Part model, mm, in its own coordinate system. A direction names the side the tool comes from. Coordinates: 2 decimals unless noted, no trailing zeros. Loops run counter-clockwise (first coordinate to the right, second up) from the corner with the lowest first, then second, coordinate; pieces in that order, holes last. Notation, with made-up numbers: M 61.25,25.25 L 110.25,25.25 A21 ccw 110.25,59.25 Z; hole C 87,56.5 d4. An arc over 180 degrees is marked long. Answer as a JSON object with one key per item and string values. Group by question number.
1. Saw through at C-C on y = -12. Write the cut outline in (x, z).
2. Saw through at A-A on x = 0. Write the cut outline in (y, z), then the cut area to 3 significant figures.
3. Saw through at D-D on x = -4.5. Write the cut outline in (y, z).
4. Drop flat-ended pins along their axis: pin 1 Ø3 at (x, y) = (-2.5, 6.5) entering from -Z; pin 2 Ø3 at (x, z) = (-7.5, 0) entering from +Y; pin 3 Ø5 at (x, y) = (-3, -13) entering from +Z; pin 4 Ø7.5 at (x, z) = (3, 1.5) entering from -Y. Give the stop position or say it passes through.
5. Drill centre lines: L1, parallel to X at y = -1.35, z = 0; L2, parallel to Z at x = 7.5, y = -2.6; L3, parallel to Y at x = 6.5, z = 2. Where is each one in solid material? Low to high.
6. Mould opens along Z. For faces 1 (the face through (0, -31, 7.7)), 2 (the face through (0, 10, 2)), 3 (the face through (7, -5, 0)) say: released by +Z, released by -Z, zero draft, split by the parting line, or undercut.
7. 3-axis set-ups, long thin cutter, end or side, ignore diameter. For faces 4 (the face through (-7.66, -45.87, -1.51)), 5 (the face through (-8, -5, 0)), 6 (the face through (7.53, -45.875, 1.783)), 7 (the face through (-7.53, -45.875, -1.783)), 8 (the face through (0, -19, -9)): which of +Z, -Z, +X, -X, +Y, -Y reach the whole face in a straight line?
from build123d import *

# Parameters (mm, degrees)
SKETCH_R                 = 10
PAD_DEPTH                = 19
SKETCH001_R              = 3.5
PAD001_DEPTH             = 3
SKETCH002_R              = 2
PAD002_DEPTH             = 14.5
SKETCH003_W              = 10
SKETCH003_H              = 5
POCKET_DEPTH             = 14.5
PAD003_DEPTH             = 25.1
SKETCH005_R              = 3.1
PAD004_DEPTH             = 2.1
SKETCH006_R              = 1
PAD005_DEPTH             = 6
PAD006_DEPTH             = 3.6
SKETCH009_R              = 0.5
POCKET001_DEPTH          = 5
POLARPATTERN_COUNT       = 2
POLARPATTERN001_COUNT    = 2
POLARPATTERN001_FACE35_R = 1
POCKET002_DEPTH          = 5
SKETCH010_R              = 1.25
POCKET003_DEPTH          = 5


with BuildPart() as part:
    # Sketch → Pad (new body)
    with BuildSketch(Plane.XZ):
        Circle(SKETCH_R)
    extrude(amount=PAD_DEPTH)

    # Sketch001 (on Face2 of Pad) → Pad001 (join)
    with BuildSketch(Plane(origin=(0, 0, 0), x_dir=(1, 0, 0), z_dir=(0, 1, 0))):
        Circle(SKETCH001_R)
    extrude(amount=PAD001_DEPTH)

    # Sketch002 (on Face5 of Pad001) → Pad002 (join)
    with BuildSketch(Plane(origin=(0, 3, 0), x_dir=(1, 0, 0), z_dir=(0, 1, 0))):
        Circle(SKETCH002_R)
    extrude(amount=PAD002_DEPTH)

    # Sketch003 (on Face7 of Pad002) → Pocket (cut)
    with BuildSketch(Plane(origin=(0, 17.5, 0), x_dir=(1, 0, 0), z_dir=(0, 1, 0))):
        with Locations((0, 4)):
            Rectangle(SKETCH003_W, SKETCH003_H)
    extrude(amount=-POCKET_DEPTH, mode=Mode.SUBTRACT)

    # Sketch004 (on Face3 of Pocket) → Pad003 (join)
    with BuildSketch(Plane.XZ.offset(19)):
        with BuildLine():
            Line((-6.689544, 7.7), (6.689544, 7.7))
            ThreePointArc((6.689544, -7.7), (10.2, 0), (6.689544, 7.7))
            Line((6.689544, -7.7), (-6.689544, -7.7))
            ThreePointArc((-6.689544, 7.7), (-10.2, 0), (-6.689544, -7.7))
        make_face()
    extrude(amount=PAD003_DEPTH)

    # Sketch005 (on Face14 of Pad003) → Pad004 (join)
    with BuildSketch(Plane.XZ.offset(44.1)):
        Circle(SKETCH005_R)
    extrude(amount=PAD004_DEPTH)

    # Sketch006 (on Face21 of Pad004) → Pad005 (join)
    with BuildSketch(Plane.XZ.offset(46.2)):
        Circle(SKETCH006_R)
    extrude(amount=PAD005_DEPTH)

    # Sketch008 (on Face14 of Pad005) → Pad006 (join)
    with BuildSketch(Plane.XZ.offset(44.1)):
        Polygon((6.603759, 1.445812), (8.483144, 2.129852), (8.58575, 1.847944), (6.706365, 1.163904), align=None)
    pad006 = extrude(amount=PAD006_DEPTH)

    # Sketch009 (on Face21 of Pad006) → Pocket001 (cut)
    with BuildSketch(Plane(origin=(0.410424, 0, -1.127631), x_dir=(0.939693, 0, 0.34202), z_dir=(0.34202, 0, -0.939693))):
        with Locations((7.689708, 46.695641)):
            Circle(SKETCH009_R)
    pocket001 = extrude(amount=-POCKET001_DEPTH, mode=Mode.SUBTRACT)

    # PolarPattern: Pad006 ×2 about axis
    polarpattern_axis = Axis((0, -44.1, 0), (0, -1, 0))
    for i in range(1, POLARPATTERN_COUNT):
        add(pad006.rotate(polarpattern_axis, i * 360 / POLARPATTERN_COUNT))

    # PolarPattern001: Pocket001 ×2 about axis
    polarpattern001_axis = Axis((0, 0, 0), (0, 1, 0))
    for i in range(1, POLARPATTERN001_COUNT):
        add(pocket001.rotate(polarpattern001_axis, i * 360 / POLARPATTERN001_COUNT), mode=Mode.SUBTRACT)

    # PolarPattern001 Face35 → Pocket002 (cut)
    with BuildSketch(Plane(origin=(0, -52.2, 0), x_dir=(-1, 0, 0), z_dir=(0, -1, 0))):
        Circle(POLARPATTERN001_FACE35_R)
    extrude(amount=-POCKET002_DEPTH, mode=Mode.SUBTRACT)

    # Sketch010 (on Face2 of Pocket002) → Pocket003 (cut)
    with BuildSketch(Plane(origin=(0, 0, 0), x_dir=(1, 0, 0), z_dir=(0, 1, 0))):
        with Locations((-7.5, 0)):
            Circle(SKETCH010_R)
        with Locations((7.5, 0)):
            Circle(SKETCH010_R)
    extrude(amount=-POCKET003_DEPTH, mode=Mode.SUBTRACT)


solid = part.part
Outcome:
{
 "1": {"outline": "C 0,0 d20"},
 "2": {"outline": "M -47.2,-1 L -46.2,-1 L -46.2,-3.1 L -44.1,-3.1 L -44.1,-7.7 L -19,-7.7 L -19,-10 L 0,-10 L 0,-3.5 L 3,-3.5 L 3,-1.5 L 17.5,-1.5 L 17.5,2 L 3,2 L 3,3.5 L 0,3.5 L 0,10 L -19,10 L -19,7.7 L -44.1,7.7 L -44.1,3.1 L -46.2,3.1 L -46.2,1 L -47.2,1 Z", "area": "853 mm²"},
 "3": {"outline": "M -44.1,-7.7 L -19,-7.7 L -19,-8.93 L 0,-8.93 L 0,8.93 L -19,8.93 L -19,7.7 L -44.1,7.7 Z"},
 "4": {"pin 1": "stops at z = -1.5", "pin 2": "stops at y = 0", "pin 3": "stops at z = 9.99", "pin 4": "stops at y = -47.7"},
 "5": {"L1": "x = -10 to -8.75, -6.25 to 6.25, 8.75 to 10", "L2": "z = -6.61 to -1.25, 1.25 to 6.61", "L3": "y = -44.1 to 0"},
 "6": {"face 1": "released by +Z", "face 2": "split by the parting line", "face 3": "undercut"},
 "7": {"face 4": "+Z, -X, -Y", "face 5": "+Y", "face 6": "+Z, -Y", "face 7": "-Z, -Y", "face 8": "-Z, +X, -X, -Y"}
}
